from build123d import *

# Parameters (mm, degrees)
F0_R     = 29.7013874084
F2_DEPTH = 38.5799203068
F1_SIZE  = 5.08
F3_R     = 20.8700317212
F3_R_2   = 17.605389727
F4_DEPTH = 28.3505246043
F6_DEPTH = 3.6485241726


with BuildPart() as f2:
    # F0 (on Front) → F2 (new body)
    with BuildSketch(Plane.XZ):
        Circle(F0_R)
    extrude(amount=F2_DEPTH)

    # F1
    f1_edges = [f2.edges().sort_by_distance(p)[0] for p in [
        (29.701387, -19.28996, 0),
        (-29.701387, 0, 0),
        (-29.701387, -38.57992, 0),
    ]]
    chamfer(f1_edges, length=F1_SIZE)

    # F3 (on face) → F4 (join)
    with BuildSketch(Plane.XZ.offset(38.5799203068)):
        Circle(F3_R)
        Circle(F3_R_2, mode=Mode.SUBTRACT)
    extrude(amount=-F4_DEPTH)

    # F5 (on face) → F6 (join)
    with BuildSketch(Plane(origin=(0, 0, 0), x_dir=(-1, 0, 0), z_dir=(0, 1, 0))):
        Polygon((-3.1568305567, 0), (-2.227387391, 0), (2.480414696, 0), (1.4310600236, 4.6359952539), (-1.5352480114, 4.6359952539), align=None)
        Polygon((2.480414696, 0), (-2.227387391, 0), (-3.1568305567, 0), (0, -3.7142876536), align=None)
        Polygon((4.7204634175, -2.7660680935), (2.480414696, 0), (0, -3.7142876536), (4.0771467611, -3.7142876536), align=None)
        Polygon((0, -3.7142876536), (-3.1568305567, 0), (-5.1875901408, -2.9743975028), (-3.672990948, -4.144215025), align=None)
    extrude(amount=F6_DEPTH)


solid = f2.part
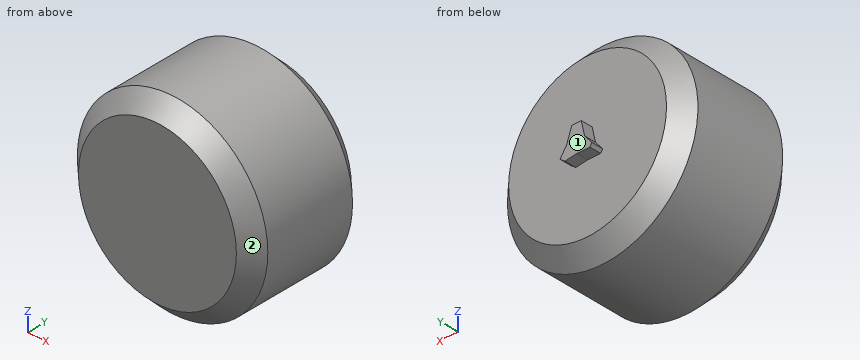
Work out the finished part from the listing and answer in its coordinate system (mm). Face numbers are marked on the shaded views. Give positions to 0.01 mm unless a question says otherwise; leave off trailing zeros. Order: outer loops, then holes, each group sorted by start corner. A loop starts at its lowest first (then second) coordinate and runs counter-clockwise, first axis right, second up. Notation, with made-up numbers: M 63.25,72 L 100.25,72 A11 cw 100.25,85 Z; hole C -38.75,-19.5 d6. An arc over 180 degrees is marked long. Return JSON: item names as keys, results as strings.
Q1. Each of these flat-tipped pins is pushed along its axis until it touches: pin 1 (12 mm diameter, centred on y = -24.5, z = -17, fed in from +X); pin 2 (8 mm diameter, centred on x = 15, y = -13, fed in from -Z); pin 3 (8 mm diameter, centred on x = 10.5, y = -9, fed in from +Z). Where does it stop, or does it pass through?
Answer below:
{"pin 1": "stops at x = 27.59", "pin 2": "stops at z = -27.59", "pin 3": "stops at z = 28.98"}
Q2. Find section A-A, the plane y = -30.5. Write down the section's boundary in (x, z).
Answer below:
{"outline": "C 0,0 d59.4"}
Q3. Find the intervals of material crossed by line 1 along Y through (x, z) = (5.5, -16.5); line 2 along X through (y, z) = (-17, 1); line 3 along Z through (x, y) = (0.5, -5), in increasing order. Write a range as [from, to].
Answer below:
{"line 1": "y = [-38.58, 0]", "line 2": "x = [-29.68, 29.68]", "line 3": "z = [-29.62, 29.62]"}
Q4. The mould has two halves that part along X. Classify the marked faces 1 and 2: pulls with the +X half, pulls with the -X half, needs draft (parallel to the pull), parting line crosses it, or undercut.
Answer below:
{"face 1": "needs draft", "face 2": "parting line crosses it"}
Q5. Find section B-B, the plane y = -3.5. Write down the section's boundary in (x, z), and give its area (3 significant figures).
Answer below:
{"outline": "C 0,0 d56.24", "area": "2,480 mm^2"}
